The listing builds one solid part. Answer for the finished solid, in the listing's coordinates (mm). A direction names the side the tool comes from. Round coordinates to 2 decimals unless told otherwise and drop trailing zeros. Write each loop counter-clockwise with the first axis right and the second up, starting at its lowest first coordinate (ties: lowest second). Pieces come first, ordered by that corner, then holes. Notation, with made-up numbers: (-22.75, 21.5) - (13.25, 21.5) arc R19 ccw to (13.25, 48.5) - close; hole circle Ø2 at (-6.5, 10.25). An arc over 180 degrees is marked (long way). Return JSON: item names as keys, results as strings. Group by question number.
(1) Section C-C, the plane z = 0.2 is taken. Write down the section's boundary in (x, y), then the cut area to 3 significant figures.
(2) Each of these flat-tipped pins is pushed along its axis until it touches: pin 1 (0.5 mm diameter, centred on y = 6, z = 1, fed in from +X); pin 2 (1.4 mm diameter, centred on x = -0.5, z = 1.5, fed in from -Y). Where does it stop, or does it pass through?
(3) Section A-A, the plane y = 0 is taken. Write down the section's boundary in (x, z).
(4) Section D-D, the plane x = -2.5 is taken. Write down the section's boundary in (y, z), then the cut area to 3 significant figures.
(5) Determine the mould class of faces 3 (the cylindrical face through (0.25, -5.995, 0.246)), 4 (the cylindrical face through (-2.579, 1.978, 0.246)), 5 (the flat face through (0, 6.6, 2)) for opening direction X: +X half, -X half, draft (parallel to the pull), parting line (faces both ways), or undercut.
(6) Section B-B, the plane x = 0 is taken. Write down the section's boundary in (y, z).
(7) Find the intervals of material crossed by line 1 along Z through (x, y) = (4.5, 0.5); line 2 along Y through (x, z) = (-1.75, 0.2); line 3 along X through (y, z) = (6.25, 0.35), in increasing order. Write a range as [from, to].
(8) Which of the six approach directions +Z, -Z, +X, -X, +Y, -Y give full straight-line access (tool end or side, diameter ignored) to faces 1 (the flat face through (3, -3, 0)), 2 (the flat face through (0, 6.1, 1))?
Autodesk Inventor part; units mm, degrees
ref_plane "YZ Plane" through (0, 0, 0) normal (1, 0, 0) x (0, 1, 0)
ref_plane "XZ Plane" through (0, 0, 0) normal (0, 1, 0) x (-1, 0, 0)
ref_plane "XY Plane" through (0, 0, 0) normal (0, 0, 1) x (1, 0, 0)
sketch "Sketch1" plane through (0, 0, 0) normal (0, 0, 1) x (1, 0, 0)
  circle A0 centre (0, 0) radius 6
  circle A1 centre (0, 0) radius 3.25
  dimension "d0" = 12
  dimension "d1" = 6.5
extrude "Extrusion1" add sketch "Sketch1" along normal blind 0.5
sketch "Sketch2" plane through (0, 0, 0) normal (1, 0, 0) x (0, 1, 0)
  line L0 (-6, 0.5) -> (6, 0.5)
  line L1 (-6, 0) -> (6, 0)
  line L2 (6, 0) -> (6, 0.5)
  line L3 (6.1, 0.6) -> (6.1, 2.4)
  line L4 (6.1, 2.4) -> (6.6, 2.4)
  line L5 (6.6, 2.4) -> (6.6, 0.6)
  arc A0 (6, 0.5) -> (6.1, 0.6) centre (6, 0.6) ccw
  arc A1 (6, 0) -> (6.6, 0.6) centre (6, 0.6) ccw
  line L6 (6, 0.5) -> (6, 0)
  point P0 (0, 0)
  dimension "d6" = 0.2
  dimension "d7" = 0.5
  dimension "d8" = 2.4
extrude "Extrusion2" add sketch "Sketch2" along normal mid plane 2
sketch "Sketch3" plane through (0, 0, 0) normal (0, 0, -1) x (-1, 0, 0)
  circle A0 centre (0, 0) radius 6
  line L0 (-1, 6.6) -> (-1, 6)
  line L1 (-1, 6) -> (0, 6)
  line L2 (0, 6) -> (1, 6)
  line L3 (1, 6) -> (1, 6.6)
  line L4 (1, 6.6) -> (-1, 6.6)
  line L5 (-1, 6) -> (-1, 5.9161)
  line L6 (1, 6) -> (1, 5.9161)
extrude "Extrusion3" add sketch "Sketch3" against normal up to surface (0.5 mm away) contours A0 L2 L6 | L5 L1 A0
properties part number "SPDT Toggle Switch Anti-Rotation Washer"
Working result:
{
 "1": {"outline": "(-1, 5.92) arc R6 ccw (long way) to (1, 5.92) - (1, 6.45) - (-1, 6.45) - close; hole circle Ø6.5 at (0, 0)", "area": "80.9 mm^2"},
 "2": {"pin 1": "stops at x = 1", "pin 2": "stops at y = 6.1"},
 "3": {"outline": "(-6, 0) - (-3.25, 0) - (-3.25, 0.5) - (-6, 0.5) - close; (3.25, 0) - (6, 0) - (6, 0.5) - (3.25, 0.5) - close"},
 "4": {"outline": "(-5.45, 0) - (-2.08, 0) - (-2.08, 0.5) - (-5.45, 0.5) - close; (2.08, 0) - (5.45, 0) - (5.45, 0.5) - (2.08, 0.5) - close", "area": "3.38 mm^2"},
 "5": {"face 3": "parting line", "face 4": "undercut", "face 5": "draft"},
 "6": {"outline": "(-6, 0) - (-3.25, 0) - (-3.25, 0.5) - (-6, 0.5) - close; (3.25, 0) - (6, 0) arc R0.6 ccw to (6.6, 0.6) - (6.6, 2.4) - (6.1, 2.4) - (6.1, 0.6) arc R0.1 cw to (6, 0.5) - (3.25, 0.5) - close"},
 "7": {"line 1": "z = [0, 0.5]", "line 2": "y = [-5.74, -2.74], [2.74, 5.74]", "line 3": "x = [-1, 1]"},
 "8": {"face 1": "-Z, +X, -X, +Y, -Y", "face 2": "+Z, +X, -X, -Y"}
}
